Check sheet for the modelled part. Datum: model origin and axes. Units: mm. A direction names the side the tool comes from. Round coordinates to 2 decimals unless told otherwise and drop trailing zeros. Loops run counter-clockwise (first coordinate to the right, second up) from the corner with the lowest first, then second, coordinate; pieces in that order, holes last. Notation, with made-up numbers: (22.25, 37) - (26.25, 37) arc R33 cw to (26.25, 74) - close; hole circle Ø7 at (-28, -13). An arc over 180 degrees is marked (long way). Return JSON: item names as keys, results as strings.
from build123d import *

# Parameters (mm, degrees)
CROQUIS1_R              = 1.5
CROQUIS1_W              = 15
CROQUIS1_H              = 2
SALIENTE_EXTRUIR1_DEPTH = 2


with BuildPart() as part:
    # Croquis1 → Saliente-Extruir1 (new, symmetric)
    with BuildSketch(Plane(origin=(0, 0, 0), x_dir=(0, 0, -1), z_dir=(1, 0, 0))):
        with BuildLine():
            Line((-10, 1), (-10, -1))
            ThreePointArc((-10, -1), (-9.414213562, -2.414213562), (-8, -3))
            Line((-8, -3), (8, -3))
            ThreePointArc((8, -3), (9.414213562, -2.414213562), (10, -1))
            Line((10, -1), (10, 1))
            ThreePointArc((10, 1), (9.414213562, 2.414213562), (8, 3))
            Line((8, 3), (3, 3))
            Line((3, 3), (3, 15))
            ThreePointArc((3, 15), (0, 18), (-3, 15))
            Line((-3, 15), (-3, 3))
            Line((-3, 3), (-8, 3))
            ThreePointArc((-8, 3), (-9.414213562, 2.414213562), (-10, 1))
        make_face()
        with Locations((0, 15)):
            Circle(CROQUIS1_R, mode=Mode.SUBTRACT)
        Rectangle(CROQUIS1_W, CROQUIS1_H, mode=Mode.SUBTRACT)
    extrude(amount=SALIENTE_EXTRUIR1_DEPTH, both=True)


solid = part.part
Q1. Sectioned sample at B-B (z = 0). Enter the section's corners in (x, y), plus the area to 3 significant figures.
Answer key:
{"outline": "(-2, -3) - (2, -3) - (2, -1) - (-2, -1) - close; (-2, 1) - (2, 1) - (2, 13.5) - (-2, 13.5) - close; (-2, 16.5) - (2, 16.5) - (2, 18) - (-2, 18) - close", "area": "64.0 mm²"}
Q2. Tool access check on faces 5 (the face through (0, 9, 3)), 6 (the face through (0, 0, -7.5)), 7 (the face through (-2, 5, 0)). Record the directions out of +Z, -Z, +X, -X, +Y, -Y that give a thin tool (end or side, any length) a straight path to the whole face; none if there is none.
Answer key:
{"face 5": "+Z, +X, -X, +Y", "face 6": "+X, -X", "face 7": "+Z, -Z, -X, +Y, -Y"}
Q3. Draft check along Z on faces 1 (the face through (0, -1, 0)), 2 (the face through (0.03, -2.4, 9.43)), 3 (the face through (0, 9, -3)), 4 (the face through (0, -3, 0)). Enter one of: released by +Z, released by -Z, zero draft, split by the parting line, or undercut.
Answer key:
{"face 1": "undercut", "face 2": "released by +Z", "face 3": "released by -Z", "face 4": "zero draft"}
Q4. Sectioned sample at A-A (x = 1.7). Enter the section's corners in (y, z).
Answer key:
{"outline": "(-3, -8) arc R2 ccw to (-1, -10) - (1, -10) arc R2 ccw to (3, -8) - (3, -3) - (15, -3) arc R3 ccw to (15, 3) - (3, 3) - (3, 8) arc R2 ccw to (1, 10) - (-1, 10) arc R2 ccw to (-3, 8) - close; hole (-1, -7.5) - (1, -7.5) - (1, 7.5) - (-1, 7.5) - close; hole circle Ø3 at (15, 0)"}
Q5. Scan lines: probe 1 along Y at (x, z) = (-1.1, 0); probe 2 along Y at (x, z) = (0.85, 5.5); probe 3 along Z at (x, y) = (-0.95, 0.75). Record each from-to range of solid material in increasing order. Write a range as [from, to].
Answer key:
{"probe 1": "y = [-3, -1], [1, 13.5], [16.5, 18]", "probe 2": "y = [-3, -1], [1, 3]", "probe 3": "z = [-10, -7.5], [7.5, 10]"}
Q6. Sectioned sample at C-C (z = -7). Enter the section's corners in (x, y), plus the area to 3 significant figures.
Answer key:
{"outline": "(-2, -3) - (2, -3) - (2, -1) - (-2, -1) - close; (-2, 1) - (2, 1) - (2, 3) - (-2, 3) - close", "area": "16.0 mm²"}
Q7. Sectioned sample at D-D (y = 14.25). Enter the section's corners in (x, z), plus the area to 3 significant figures.
Answer key:
{"outline": "(-2, -3) - (2, -3) - (2, -1.3) - (-2, -1.3) - close; (-2, 1.3) - (2, 1.3) - (2, 3) - (-2, 3) - close", "area": "13.6 mm²"}
Q8. Depth check by flat-ended pin: P1, Ø1, axis at x = 1, y = 14, coming from the -Z side; P2, Ø2, axis at x = 0, z = 4.5, coming from the +Y side. Enter the tip coordinate at first touch or a pass-through.
Answer key:
{"P1": "stops at z = -3", "P2": "stops at y = 3"}
